Source: CAD feature listing. Evaluate the final solid. Frame: model axes, mm. A direction names the side the tool comes from. Give positions to 0.01 mm unless a question says otherwise; leave off trailing zeros. Write each loop counter-clockwise with the first axis right and the second up, starting at its lowest first coordinate (ties: lowest second). Pieces come first, ordered by that corner, then holes. Notation, with made-up numbers: M 49,-37 L 102,-37 A28 ccw 102,-1 Z; hole C 79.5,30.5 d2. An arc over 180 degrees is marked long. Return JSON: item names as keys, results as strings.
```python
from build123d import *

# Parameters (mm, degrees)
SKETCH_1_R          = 31.75
EXTRUDE_1_DEPTH     = 14.5
CHAMFER_1_SIZE      = 1
SKETCH_3_R          = 30.75
SKETCH_2_R          = 22
SKETCH_4_R          = 6.3
CUT_EXTRUDE_1_DEPTH = 48.836962696
CUT_EXTRUDE_2_DEPTH = 5
SKETCH_6_R          = 27.5
CUT_EXTRUDE_3_DEPTH = 11.5
M3X0_51_D           = 2.5
SKETCH_11_R         = 10
SKETCH_11_R_2       = 6.3
EXTRUDE_2_DEPTH     = 11.5


with BuildPart() as part:
    # Эскиз1 → Бобышка-Вытянуть1 (new body)
    with BuildSketch(Plane.XY):
        with Locations(Location((0, 0, 0), (0, 0, 180))):
            Circle(SKETCH_1_R)
    extrude(amount=EXTRUDE_1_DEPTH)

    # Фаска1
    chamfer_1_edges = [part.edges().sort_by_distance(p)[0] for p in [
        (31.75, 0, 14.5),
    ]]
    chamfer(chamfer_1_edges, length=CHAMFER_1_SIZE)

    # Эскиз3 → По сечениям3 section 0
    with BuildSketch(Plane.XY.offset(14.5)):
        Circle(SKETCH_3_R)
    # Эскиз2 → По сечениям3 section 1
    with BuildSketch(Plane.XY.offset(16.5)):
        Circle(SKETCH_2_R)
    loft()

    # Эскиз4 → Вырез-Вытянуть1 (cut, through all)
    with BuildSketch(Plane.XY.offset(16.5)):
        Circle(SKETCH_4_R)
    extrude(amount=-CUT_EXTRUDE_1_DEPTH, mode=Mode.SUBTRACT)

    # Эскиз5 → Вырез-Вытянуть2 (cut)
    with BuildSketch(Plane.XY.offset(16.5)):
        with BuildLine():
            Line((-8.660254038, 15), (-15.875, 27.49630657))
            ThreePointArc((-15.875, 27.49630657), (0, 31.75), (15.875, 27.49630657))
            Line((15.875, 27.49630657), (8.660254038, 15))
            ThreePointArc((8.660254038, 15), (0, 10), (-8.660254038, 15))
        make_face()
        with BuildLine():
            Line((15, 8.660254038), (27.49630657, 15.875))
            ThreePointArc((27.49630657, 15.875), (31.75, 0), (27.49630657, -15.875))
            Line((27.49630657, -15.875), (15, -8.660254038))
            ThreePointArc((15, -8.660254038), (10, 0), (15, 8.660254038))
        make_face()
        with BuildLine():
            Line((8.660254038, -15), (15.875, -27.49630657))
            ThreePointArc((15.875, -27.49630657), (0, -31.75), (-15.875, -27.49630657))
            Line((-15.875, -27.49630657), (-8.660254038, -15))
            ThreePointArc((-8.660254038, -15), (0, -10), (8.660254038, -15))
        make_face()
        with BuildLine():
            Line((-15, -8.660254038), (-27.49630657, -15.875))
            ThreePointArc((-27.49630657, -15.875), (-31.75, 0), (-27.49630657, 15.875))
            Line((-27.49630657, 15.875), (-15, 8.660254038))
            ThreePointArc((-15, 8.660254038), (-10, 0), (-15, -8.660254038))
        make_face()
    extrude(amount=-CUT_EXTRUDE_2_DEPTH, mode=Mode.SUBTRACT)

    # Эскиз6 → Вырез-Вытянуть3 (cut)
    with BuildSketch(Plane(origin=(0, 0, 0), x_dir=(-1, 0, 0), z_dir=(0, 0, -1))):
        Circle(SKETCH_6_R)
    extrude(amount=-CUT_EXTRUDE_3_DEPTH, mode=Mode.SUBTRACT)

    # Отверстие обработанное метчиком M3x0.51 (through all)
    with Locations(Plane.XY.offset(16.5)):
        with Locations((-8.838834765, 8.838834765), (-8.838834765, -8.838834765), (8.838834765, -8.838834765), (8.838834765, 8.838834765)):
            Hole(M3X0_51_D / 2)

    # Эскиз11 → Бобышка-Вытянуть2 (add)
    with BuildSketch(Plane(origin=(0, 0, 11.5), x_dir=(-1, 0, 0), z_dir=(0, 0, -1))):
        with Locations(Location((0, 0, 0), (0, 0, 180))):
            Circle(SKETCH_11_R)
        with Locations(Location((0, 0, 0), (0, 0, 180))):
            Circle(SKETCH_11_R_2, mode=Mode.SUBTRACT)
    extrude(amount=EXTRUDE_2_DEPTH)


solid = part.part
```
1) Cut plane B-B, the plane y = -3.5. Return the cut outline in (x, z).
Numbers:
{"outline": "M -31.56,0 L -27.28,0 L -27.28,11.5 L -31.56,11.5 Z; M -10.63,11.5 L -9.37,11.5 L -9.37,0 L -5.24,0 L -5.24,16.5 L -10.63,16.5 Z; M 5.24,0 L 9.37,0 L 9.37,11.5 L 10.63,11.5 L 10.63,16.5 L 5.24,16.5 Z; M 27.28,0 L 31.56,0 L 31.56,11.5 L 27.28,11.5 Z"}
2) Line query: line 1 (Y direction, x = -1, z = 1.25); line 2 (Y direction, x = 7.5, z = 5.25); line 3 (Z direction, x = -11, y = 9.5). Output: solid intervals per line, ascending. Write a range as [from, to].
Numbers:
{"line 1": "y = [-31.73, -27.48], [-9.95, -6.22], [6.22, 9.95], [27.48, 31.73]", "line 2": "y = [-30.85, -26.46], [-6.61, 6.61], [26.46, 30.85]", "line 3": "z = [11.5, 16.5]"}
3) Cut plane A-A, the plane z = 8. Return the cut outline in (x, y), then the cut area to 3 significant figures.
Numbers:
{"outline": "C 0,0 d63.5; C 0,0 d20; hole C 0,0 d55; hole C 0,0 d12.6", "area": "981 mm²"}
4) Draft query along X for faces 1 (the face through (-21.85, 22.02, 14.23)), 2 (the face through (0, 7, 0)), 3 (the face through (0, 10, 14)), 4 (the face through (21.161, 12.217, 13.479)). Return one class per face: released by +X, released by -X, zero draft, split by the parting line, or undercut.
Numbers:
{"face 1": "released by -X", "face 2": "zero draft", "face 3": "undercut", "face 4": "released by +X"}
5) Set-up query: faces 5 (the face through (10, 0, 14)), 6 (the face through (-21.34, 12.32, 13.48)), 7 (the face through (-7.918, 9.684, 13.965)), 8 (the face through (-12.32, -21.34, 13.48)), 9 (the face through (14, 14, 11.5)). Return all of +Z, -Z, +X, -X, +Y, -Y with unobstructed straight access to the full face (end or side cutting, diameter ignored); none if empty.
Numbers:
{"face 5": "+Z, -Z, +X", "face 6": "+Z, -X", "face 7": "+Z, -Z", "face 8": "+Z, -Y", "face 9": "-Z"}
6) Contact query for flat-ended pins moving along their axis: pin 1 Ø2.5 at (x, y) = (28.5, -2) entering from +Z; pin 2 Ø6 at (y, z) = (5, 4.5) entering from -X; pin 3 Ø4 at (x, z) = (-17.5, 12.5) entering from +Y. Output: stop coordinate, or through.
Numbers:
{"pin 1": "stops at z = 11.5", "pin 2": "stops at x = -31.69", "pin 3": "stops at y = 27.56"}
